from build123d import *

# Parameters (mm, degrees)
F0_W     = 43.6
F0_H     = 43.6
F2_DEPTH = 3
F3_R     = 1.65
F4_DEPTH = 25
F1_W     = 43.6
F1_H     = 43.6
F5_DEPTH = 35
F7_DEPTH = 25


with BuildPart() as f2:
    # F0 (on Top) → F2 (new body)
    with BuildSketch(Plane.XY):
        with Locations((-1.601375, 0.614843)):
            Rectangle(F0_W, F0_H)
    extrude(amount=F2_DEPTH)

    # F3 (on face) → F4 (cut)
    with BuildSketch(Plane.XY.offset(3)):
        with Locations((-20.051375, 19.264843)):
            Circle(F3_R)
        with Locations((16.848625, 19.264843)):
            Circle(F3_R)
        with Locations((16.848625, -18.035157)):
            Circle(F3_R)
        with Locations((-20.051375, -18.035157)):
            Circle(F3_R)
    extrude(amount=-F4_DEPTH, mode=Mode.SUBTRACT)

    # F1 (on Top) → F5 (join)
    with BuildSketch(Plane.XY):
        Polygon((20.198625, 26.914843), (-23.401375, 26.914843), (-27.901375, 26.914843), (-27.901375, 22.414843), (-27.901375, -21.185157), (-27.901375, -25.685157), (-23.401375, -25.685157), (20.198625, -25.685157), (24.698625, -25.685157), (24.698625, -21.185157), (24.698625, 22.414843), (24.698625, 26.914843), align=None)
        with Locations((-1.601375, 0.614843)):
            Rectangle(F1_W, F1_H, mode=Mode.SUBTRACT)
    extrude(amount=F5_DEPTH)

    # F6 (on face) → F7 (cut)
    with BuildSketch(Plane(origin=(0, 26.914843, 0), x_dir=(-1, 0, 0), z_dir=(0, 1, 0))):
        Polygon((-5.790295, 21.375465), (-4.23457, 23.161669), (-5.003605, 25.402069), (-7.328367, 25.856265), (-8.884092, 24.070061), (-8.115056, 21.829661), align=None)
        Polygon((-8.115056, 10.929661), (-5.790295, 10.475465), (-4.23457, 12.261669), (-5.003605, 14.502069), (-7.328367, 14.956265), (-8.884092, 13.170061), align=None)
        Polygon((0.1, 21.6), (2.424761, 21.145804), (3.980487, 22.932009), (3.211451, 25.172409), (0.88669, 25.626604), (-0.669036, 23.8404), align=None)
        Polygon((0.1, 10.7), (2.424761, 10.245804), (3.980487, 12.032009), (3.211451, 14.272409), (0.88669, 14.726604), (-0.669036, 12.9404), align=None)
        Polygon((8.315056, 21.370339), (10.639818, 20.916144), (12.195543, 22.702348), (11.426507, 24.942748), (9.101746, 25.396944), (7.546021, 23.610739), align=None)
        Polygon((8.315056, 10.470339), (10.639818, 10.016144), (12.195543, 11.802348), (11.426507, 14.042748), (9.101746, 14.496944), (7.546021, 12.710739), align=None)
    extrude(amount=-F7_DEPTH, mode=Mode.SUBTRACT)


solid = f2.part
Could you check a few things on this model? Use its own coordinates, in mm. A direction names the side the tool comes from. Give positions to 0.01 mm unless a question says otherwise; leave off trailing zeros. Write each loop counter-clockwise with the first axis right and the second up, starting at its lowest first coordinate (ties: lowest second). Pieces come first, ordered by that corner, then holes. Notation, with made-up numbers: (60, 69.25) -> (75, 69.25) arc R30 cw to (75, 100.25) -> close; hole circle Ø10 at (56, -2.5). An arc over 180 degrees is marked (long way). Write each question's results on one line, items separated by ' | '. Start each with the question number.
Q1. Suppose I cut it at C-C, the plane y = 7.5. List the corners of the cut face in (x, z) for me, and give its area (3 significant figures).
Q2. I'm going to push flat-ended pins straight in: pin 1 Ø12 at (x, y) = (15, 11.5) entering from +Z; pin 2 Ø3 at (x, y) = (-20.05, 19.26) entering from +Z; pin 3 Ø22 at (x, y) = (-5.5, -1.5) entering from +Z. Where does each tip first touch, or does it pass through?
Q3. Suppose I cut it at B-B, the plane z = 7. List the corners of the cut face in (x, y) for me.
Q4. Suppose I cut it at D-D, the plane x = 17.5. List the corners of the cut face in (y, z) for me, and give its area (3 significant figures).
Q5. We'd pull the mould along Y, two halves only. Please class faces 1 (the face through (-23.401, 0, 19)), 2 (the face through (17.736, -16.644, 1.521)), 3 (the face through (-7.925, 24.696, 11.606)): +Y half, -Y half, draft (parallel to the pull), parting line (faces both ways), or undercut.
Q6. Suppose I cut it at A-A, the plane x = 3.5. List the corners of the cut face in (y, z) for me, and give its area (3 significant figures).
Q7. Which directions (+Z, -Z, +X, -X, +Y, -Y) give clear straight access to the entire face, cutting with the end or side of a thin tool? Please do faces 4 (the face through (24.699, 0, 17)), 5 (the face through (-2.065, 24.696, 25.396)), 6 (the face through (-2, 22.415, 19)).
Q8. I need wall thicknesses on probe 1 along Y at (x, z) = (10.5, 23); probe 2 along X at (y, z) = (12.5, 27); probe 3 along Z at (x, y) = (11, 16). Which ranges of each line are inside material? Lowest first, please.
Outcome:
1) outline: (-27.9, 0) -> (24.7, 0) -> (24.7, 35) -> (20.2, 35) -> (20.2, 3) -> (-23.4, 3) -> (-23.4, 35) -> (-27.9, 35) -> close | area: 446 mm2
2) pin 1: z = 35 | pin 2: through | pin 3: z = 3
3) outline: (-27.9, -25.69) -> (24.7, -25.69) -> (24.7, 26.91) -> (-27.9, 26.91) -> close; hole (-23.4, -21.19) -> (20.2, -21.19) -> (20.2, 22.41) -> (-23.4, 22.41) -> close
4) outline: (-25.69, 0) -> (-19.55, 0) -> (-19.55, 3) -> (-21.19, 3) -> (-21.19, 35) -> (-25.69, 35) -> close; (-16.52, 0) -> (17.75, 0) -> (17.75, 3) -> (-16.52, 3) -> close; (20.78, 0) -> (26.91, 0) -> (26.91, 35) -> (22.41, 35) -> (22.41, 3) -> (20.78, 3) -> close | area: 428 mm2
5) face 1: undercut | face 2: undercut | face 3: draft
6) outline: (-25.69, 0) -> (26.91, 0) -> (26.91, 35) -> (22.41, 35) -> (22.41, 3) -> (-21.19, 3) -> (-21.19, 35) -> (-25.69, 35) -> close | area: 446 mm2
7) face 4: +Z, -Z, +X, +Y, -Y | face 5: +Y | face 6: +Z
8) probe 1: -25.69 to -21.19, 22.41 to 26.91 | probe 2: -27.9 to -23.4, 20.2 to 24.7 | probe 3: 0 to 3
